For this review, take the finished solid that the model builds, in its own axes (mm). A direction names the side the tool comes from. Give positions to 0.01 mm unless a question says otherwise; leave off trailing zeros. Loops run counter-clockwise (first coordinate to the right, second up) from the corner with the lowest first, then second, coordinate; pieces in that order, holes last. Notation, with made-up numbers: M 86.25,3.5 L 103.25,3.5 A8 cw 103.25,11.5 Z; hole C -25,8.5 d5. An arc over 180 degrees is marked long. Use CSV: the item, a comma, the result in double quotes. Start each with the question number.
1. To check wall thickness, follow line 1 (Y direction, x = 0, z = 18.5); line 2 (X direction, y = 0, z = 38); line 3 (Z direction, x = 4.25, y = 2.75). State the ranges of each line that lie inside material, in increasing order. Write a range as [from, to].
2. Take a section at D-D, the plane x = 3.25. Write out the cut boundary in (y, z).
3. The part is to be moulded in two halves that separate along X. For faces 4 (the face through (-2, 0, 40)), 5 (the face through (-2.17, -9.76, 4.93)), 6 (the face through (-2.5, -10, 40.2)), say which applies: pulls with the +X half, pulls with the -X half, needs draft (parallel to the pull), parting line crosses it, or undercut.
4. Take a section at B-B, the plane y = 0. Write out the cut boundary in (x, z), and give its area (3 significant figures).
5. Take a section at A-A, the plane x = 0. Write out the cut boundary in (y, z).
6. Tool access review of faces 1 (the face through (-3, 0, 40)), 2 (the face through (-2.3, 0.8, 60)), 3 (the face through (-2.5, 0.1, 19.8)): name each direction out of +Z, -Z, +X, -X, +Y, -Y from which nothing blocks a thin tool from reaching the whole face with its end or side.
7. Insertion check: P1, Ø12, axis at x = -0.5, y = -4, coming from the -Z side; P2, Ø12, axis at x = 6, z = 18, coming from the +Y side; P3, Ø1, axis at y = 1.5, z = 12.5, coming from the -X side; P4, Ø10, axis at y = -1.5, z = 36.5, coming from the -X side. Each pin has a flat end and moves straight along its axis. Give the tip position at first contact, or say it passes through.
8. Take a section at C-C, the plane z = 26.5. Write out the cut boundary in (x, y), and give its area (3 significant figures).
from build123d import *

# Parameters (mm, degrees)
SKETCH_1_R          = 10
SKETCH_1_R_2        = 2.6
EXTRUDE_1_DEPTH     = 10
SKETCH_2_R          = 4.6
SKETCH_2_R_2        = 2.6
EXTRUDE_2_DEPTH     = 50
CUT_EXTRUDE_1_DEPTH = 41
SKETCH_5_W          = 1
SKETCH_5_H          = 20
EXTRUDE_3_DEPTH     = 40.2


with BuildPart() as part:
    # 草图1 → 凸台-拉伸1 (new body)
    with BuildSketch(Plane.XY):
        Circle(SKETCH_1_R)
        Circle(SKETCH_1_R_2, mode=Mode.SUBTRACT)
    extrude(amount=EXTRUDE_1_DEPTH)

    # 草图2 → 凸台-拉伸2 (add)
    with BuildSketch(Plane.XY.offset(10)):
        Circle(SKETCH_2_R)
        Circle(SKETCH_2_R_2, mode=Mode.SUBTRACT)
    extrude(amount=EXTRUDE_2_DEPTH)

    # 草图3 → 切除-拉伸1 (cut)
    with BuildSketch(Plane.XY.offset(60)):
        with BuildLine():
            Line((-2, 4.142463035), (-2, -4.142463035))
            ThreePointArc((-2, -4.142463035), (-4.6, 0), (-2, 4.142463035))
        make_face()
    extrude(amount=-CUT_EXTRUDE_1_DEPTH, mode=Mode.SUBTRACT)

    # 草图5 → 凸台-拉伸3 (add)
    with BuildSketch(Plane.XY.offset(60)):
        with Locations((-2.5, 0)):
            Rectangle(SKETCH_5_W, SKETCH_5_H)
    extrude(amount=-EXTRUDE_3_DEPTH)


solid = part.part
Result set:
1,line 1,"[-4.6, -2.6], [2.6, 4.6]"
1,line 2,"[-3, -2], [2.6, 4.6]"
1,line 3,"[0, 10]"
2,outline,"M -9.46,0 L 9.46,0 L 9.46,10 L 3.26,10 L 3.26,60 L -3.26,60 L -3.26,10 L -9.46,10 Z"
3,face 4,"undercut"
3,face 5,"parting line crosses it"
3,face 6,"needs draft"
4,outline,"M -10,0 L -2.6,0 L -2.6,19 L -4.6,19 L -4.6,10 L -10,10 Z; M -3,19.8 L -2,19.8 L -2,60 L -3,60 Z; M 2.6,0 L 10,0 L 10,10 L 4.6,10 L 4.6,60 L 2.6,60 Z"
4,area,"306 mm2"
5,outline,"M -10,0 L -2.6,0 L -2.6,60 L -4.6,60 L -4.6,10 L -10,10 Z; M 2.6,0 L 10,0 L 10,10 L 4.6,10 L 4.6,60 L 2.6,60 Z"
6,face 1,"+Z, -X, +Y, -Y"
6,face 2,"+Z, +X, -X, +Y, -Y"
6,face 3,"-X, +Y, -Y"
7,P1,"z = 0"
7,P2,"y = 4.6"
7,P3,"x = -4.49"
7,P4,"x = -3"
8,outline,"M -3,-10 L -2,-10 L -2,-4.14 A4.6 ccw long -2,4.14 L -2,10 L -3,10 Z; hole M -2,-1.66 A2.6 ccw long -2,1.66 Z"
8,area,"51.2 mm2"
